```python
from build123d import *

# Parameters (mm, degrees)
SKETCH1_R           = 2
BOSS_EXTRUDE1_DEPTH = 5
SKETCH2_W           = 0.1
SKETCH2_H           = 5
CUT_EXTRUDE1_DEPTH  = 3
SKETCH3_W           = 0.1
SKETCH3_H           = 5
CUT_EXTRUDE2_DEPTH  = 3
SKETCH4_W           = 5
SKETCH4_H           = 5
CUT_EXTRUDE3_DEPTH  = 2.5
FILLET1_R           = 10


with BuildPart() as part:
    # Sketch1 → Boss-Extrude1 (new body)
    with BuildSketch(Plane.XY):
        with BuildLine():
            Line((1, 0), (17, 0))
            ThreePointArc((17, 0), (24.071067812, -2.928932188), (27, -10))
            Line((27, -10), (27, -10.164726931))
            Line((27, -10.164726931), (27, -46.377180563))
            Line((27, -46.377180563), (26.694646109, -58.493944172))
            Line((26.694646109, -58.493944172), (26.694646109, -64.399649032))
            Line((26.694646109, -64.399649032), (26.694646109, -64.648499642))
            Line((26.694646109, -64.648499642), (45.291824906, -83.245678439))
            ThreePointArc((45.291824906, -83.245678439), (45.524094874, -83.868523218), (45.205420336, -84.451902592))
            Line((45.205420336, -84.451902592), (44.749875598, -84.792762343))
            ThreePointArc((44.749875598, -84.792762343), (44.625232832, -84.869323208), (44.488733304, -84.921908985))
            Line((44.488733304, -84.921908985), (38.461997774, -86.629961997))
            ThreePointArc((38.461997774, -86.629961997), (38.153804902, -86.655191857), (37.859066622, -86.561657168))
            ThreePointArc((37.859066622, -86.561657168), (36.668252624, -85.793859327), (35.597906198, -84.865468229))
            Line((35.597906198, -84.865468229), (21.037791859, -70.305353891))
            Line((21.037791859, -70.305353891), (16.801941123, -70.305353891))
            Line((16.801941123, -70.305353891), (1, -70.305353891))
            ThreePointArc((1, -70.305353891), (0.292893219, -70.012460672), (0, -69.305353891))
            Line((0, -69.305353891), (0, -64))
            ThreePointArc((0, -64), (0.292893219, -63.292893219), (1, -63))
            Line((1, -63), (10.539737479, -63))
            ThreePointArc((10.539737479, -63), (17.229153259, -60.229153259), (20, -53.539737479))
            Line((20, -53.539737479), (20, -16.460262521))
            ThreePointArc((20, -16.460262521), (17.229153259, -9.770846741), (10.539737479, -7))
            Line((10.539737479, -7), (1, -7))
            ThreePointArc((1, -7), (0.292893219, -6.707106781), (0, -6))
            Line((0, -6), (0, -1))
            ThreePointArc((0, -1), (0.292893219, -0.292893219), (1, 0))
        make_face()
        with Locations((35.887034264, -79.497742046)):
            Circle(SKETCH1_R, mode=Mode.SUBTRACT)
    extrude(amount=BOSS_EXTRUDE1_DEPTH)

    # Sketch2 → Cut-Extrude1 (cut)
    with BuildSketch(Plane(origin=(0, -63, 0), x_dir=(1, 0, 0), z_dir=(0, 1, 0))):
        with Locations((6.05, -2.5)):
            Rectangle(SKETCH2_W, SKETCH2_H)
    extrude(amount=-CUT_EXTRUDE1_DEPTH, mode=Mode.SUBTRACT)

    # Sketch3 → Cut-Extrude2 (cut)
    with BuildSketch(Plane.XZ.offset(7)):
        with Locations((6.05, 2.5)):
            Rectangle(SKETCH3_W, SKETCH3_H)
    extrude(amount=-CUT_EXTRUDE2_DEPTH, mode=Mode.SUBTRACT)

    # Sketch4 → Cut-Extrude3 (cut)
    with BuildSketch(Plane(origin=(25.586241806, -90.279113957, 0), x_dir=(0.962106712, 0.272673201, 0), z_dir=(0.272673201, -0.962106712, 0))):
        with Locations((16.490695772, 2.5)):
            Rectangle(SKETCH4_W, SKETCH4_H)
    extrude(amount=-CUT_EXTRUDE3_DEPTH, mode=Mode.SUBTRACT)

    # Fillet1
    fillet1_edges = [part.edges().sort_by_distance(p)[0] for p in [
        (26.694646109, -64.648499642, 2.5),
        (21.037791859, -70.305353891, 2.5),
    ]]
    fillet(fillet1_edges, radius=FILLET1_R)


solid = part.part
```
Source: CAD feature listing. Evaluate the final solid. Frame: model axes, mm. A direction names the side the tool comes from. Round coordinates to 2 decimals unless told otherwise and drop trailing zeros. Loops run counter-clockwise (first coordinate to the right, second up) from the corner with the lowest first, then second, coordinate; pieces in that order, holes last. Notation, with made-up numbers: M 56,75.25 L 106,75.25 A24 ccw 106,100.25 Z; hole C 26.25,7 d11. An arc over 180 degrees is marked long. Use a Markdown table: item, result. Add a question column.
1. Cut plane D-D, the plane x = 28.5. Output: boundary loops of the cut face in (y, z), and give its area (3 significant figures).
2. Contact query for flat-ended pins moving along their axis: pin 1 (10 mm diameter, centred on x = 34, y = -23.5, fed in from +Z); pin 2 (2 mm diameter, centred on x = 8.5, z = 3, fed in from -Y); pin 3 (1 mm diameter, centred on x = 19.5, y = -59, fed in from -Z); pin 4 (3 mm diameter, centred on y = -35.5, z = 4.5, fed in from -X). Output: stop coordinate, or through.
3. Cut plane B-B, the plane y = -65. Output: boundary loops of the cut face in (x, z).
4. Pull-direction query (X, two-part tool) for faces 1 (the flat face through (43.521, -83.915, 2.465)), 2 (the flat face through (21, -43, 5)), 3 (the cylindrical face through (17.3, -9.84, 2.46)); classes: +X half, -X half, draft (parallel to the pull), parting line (faces both ways), or undercut.
5. Cut plane C-C, the plane y = -36. Output: boundary loops of the cut face in (x, z).
6. Cut plane A-A, the plane x = 3. Output: boundary loops of the cut face in (y, z), and give its area (3 significant figures).
7. Set-up query: faces 4 (the cylindrical face through (37.795, -78.897, 2.465)), 5 (the cylindrical face through (17.16, -60.3, 2.46)), 6 (the flat face through (9, -70.305, 2)). Return all of +Z, -Z, +X, -X, +Y, -Y with unobstructed straight access to the full face (end or side cutting, diameter ignored); none if empty.
8. Ray query, line 1 along Y through (x, z) = (5.5, 3.9); line 2 along X through (y, z) = (-26, 3.1); line 3 along Y through (x, z) = (36.5, 1.05). Return the intervals inside material, ascending. Write a range as [from, to].
Solution:
| question | item | result |
|---|---|---|
| 1 | outline | M -77.77,0 L -66.24,0 L -66.24,5 L -77.77,5 Z |
| 1 | area | 57.6 mm2 |
| 2 | pin 1 | passes through |
| 2 | pin 2 | stops at y = -70.31 |
| 2 | pin 3 | stops at z = 0 |
| 2 | pin 4 | stops at x = 20 |
| 3 | outline | M 0,0 L 6,0 L 6,5 L 0,5 Z; M 6.1,0 L 27.76,0 L 27.76,5 L 6.1,5 Z |
| 4 | face 1 | undercut |
| 4 | face 2 | draft |
| 4 | face 3 | -X half |
| 5 | outline | M 20,0 L 27,0 L 27,5 L 20,5 Z |
| 6 | outline | M -70.31,0 L -63,0 L -63,5 L -70.31,5 Z; M -7,0 L 0,0 L 0,5 L -7,5 Z |
| 6 | area | 71.5 mm2 |
| 7 | face 4 | +Z, -Z |
| 7 | face 5 | +Z, -Z, -X |
| 7 | face 6 | +Z, -Z, -X, -Y |
| 8 | line 1 | y = [-70.31, -63], [-7, 0] |
| 8 | line 2 | x = [20, 27] |
| 8 | line 3 | y = [-85.66, -81.4], [-77.59, -74.45] |
